Work out the finished part from the listing and answer in its coordinate system (mm). A direction names the side the tool comes from. Give positions to 0.01 mm unless a question says otherwise; leave off trailing zeros. Loops run counter-clockwise (first coordinate to the right, second up) from the corner with the lowest first, then second, coordinate; pieces in that order, holes last. Notation, with made-up numbers: M -7.75,-26 L 10.25,-26 A32 cw 10.25,3 Z; hole C 65.25,41.25 d3. An arc over 180 degrees is marked long. Use a Markdown table: item, result.
```python
from build123d import *

# Parameters (mm, degrees)
SKETCH_R              = 50
PAD_DEPTH             = 3
SKETCH004_R           = 5.2
POCKET001_DEPTH       = 3.001
POCKET002_DEPTH       = 3.001
SKETCH006_R           = 50
SKETCH006_R_2         = 46
PAD001_DEPTH          = 17.5
POCKET003_DEPTH       = 3
POLARPATTERN001_COUNT = 3
PAD002_DEPTH          = 2.8
POLARPATTERN002_COUNT = 3


with BuildPart() as part:
    # Sketch → Pad (new body)
    with BuildSketch(Plane.XY):
        Circle(SKETCH_R)
    extrude(amount=PAD_DEPTH)

    # Sketch004 (on DatumPlane) → Pocket001 (cut, through all)
    with BuildSketch(Plane.XY.offset(3)):
        Circle(SKETCH004_R)
    extrude(amount=-POCKET001_DEPTH, mode=Mode.SUBTRACT)

    # Sketch005 → Pocket002 (cut, through all)
    with BuildSketch(Plane.XY):
        with BuildLine():
            ThreePointArc((12.9390240745, -44.1427418269), (23, -39.8371685741), (31.7592237776, -33.2768944622))
            Line((16.9700186383, -18.3580627359), (31.7592237776, -33.2768944622))
            ThreePointArc((7.4135393744, -23.8754986114), (12.5, -21.6506350946), (16.9700186383, -18.3580627359))
            Line((12.9390240745, -44.1427418269), (7.4135393744, -23.8754986114))
        make_face()
    extrude(amount=POCKET002_DEPTH, mode=Mode.SUBTRACT)

    # Sketch006 → Pad001 (join)
    with BuildSketch(Plane.XY):
        Circle(SKETCH006_R)
        Circle(SKETCH006_R_2, mode=Mode.SUBTRACT)
    extrude(amount=-PAD001_DEPTH)

    # Sketch007 (on DatumPlane) → Pocket003 (cut)
    with BuildSketch(Plane.XY.offset(3)):
        with BuildLine():
            ThreePointArc((-45.3011566386, 7.9878161727), (-46, 0), (-45.3011566386, -7.9878161727))
            Line((-45.3011566386, -7.9878161727), (-47.2707721446, -8.335112528))
            ThreePointArc((-47.2707721446, 8.335112528), (-48, 0), (-47.2707721446, -8.335112528))
            Line((-47.2707721446, 8.335112528), (-45.3011566386, 7.9878161727))
        make_face()
    pocket003 = extrude(amount=-POCKET003_DEPTH, mode=Mode.SUBTRACT)

    # PolarPattern001: Pocket003 ×3 about axis
    polarpattern001_axis = Axis((0, 0, 3), (0, 0, 1))
    for i in range(1, POLARPATTERN001_COUNT):
        add(pocket003.rotate(polarpattern001_axis, i * 360 / POLARPATTERN001_COUNT), mode=Mode.SUBTRACT)

    # Sketch008 (on DatumPlane) → Pad002 (join)
    with BuildSketch(Plane.XY.offset(-17.5)):
        with BuildLine():
            ThreePointArc((45.3691376707, -7.5921898696), (46, 0), (45.3691376707, 7.5921898696))
            Line((47.1444517535, 7.8892755601), (45.3691376707, 7.5921898696))
            ThreePointArc((47.1444517535, -7.8892755601), (47.8, 0), (47.1444517535, 7.8892755601))
            Line((45.3691376707, -7.5921898696), (47.1444517535, -7.8892755601))
        make_face()
    pad002 = extrude(amount=-PAD002_DEPTH)

    # PolarPattern002: Pad002 ×3 about axis
    polarpattern002_axis = Axis((0, 0, -17.5), (0, 0, 1))
    for i in range(1, POLARPATTERN002_COUNT):
        add(pad002.rotate(polarpattern002_axis, i * 360 / POLARPATTERN002_COUNT))


solid = part.part
```
(1) Which of the six approach directions +Z, -Z, +X, -X, +Y, -Y give full straight-line access (tool end or side, diameter ignored) to faces 1 (the flat face through (10, 1, 0)), 2 (the cylindrical face through (23.898, -41.628, 1.521)), 3 (the flat face through (24.26, -25.71, 1.48))?
Entries:
| item | result |
|---|---|
| face 1 | -Z |
| face 2 | +Z |
| face 3 | +Z, -Z |
(2) Given P1, Ø10, axis at y = 27.5, z = -7, coming from the -X side; P2, Ø12, axis at x = -20, z = -7.5, coming from the -Y side; P3, Ø3, axis at x = 7, z = -6, coming from the +Y side, each flat-ended and moving along its own axis, determine where each tip first touches the part or whether it passes through.
Entries:
| item | result |
|---|---|
| P1 | stops at x = -44.65 |
| P2 | stops at y = -48 |
| P3 | stops at y = 49.7 |
(3) A cutting plane is placed at B-B (x = 0). Write down the section's boundary in (y, z), and give its area (3 significant figures).
Entries:
| item | result |
|---|---|
| outline | M -50,-17.5 L -46,-17.5 L -46,0 L -5.2,0 L -5.2,3 L -50,3 Z; M 5.2,0 L 46,0 L 46,-17.5 L 50,-17.5 L 50,3 L 5.2,3 Z |
| area | 409 mm² |
(4) The mould has two halves that part along Y. Classify faces 4 (the cylindrical face through (47.8, -0.1, -18.9)), 5 (the cylindrical face through (-23.804, 41.451, -18.88)), 6 (the flat face through (-47, 0, 0)), 7 (the cylindrical face through (-24, -41.34, -18.88)): released by +Y, released by -Y, zero draft, split by the parting line, or undercut.
Entries:
| item | result |
|---|---|
| face 4 | split by the parting line |
| face 5 | released by +Y |
| face 6 | undercut |
| face 7 | released by -Y |
(5) Consider probe 1 along Y at (x, z) = (0, 2.35); probe 2 along Y at (x, z) = (0, -11.75); probe 3 along X at (y, z) = (27.5, -11.5). Determine where each line is inside the solid, lowest interval first. Write a range as [from, to].
Entries:
| item | result |
|---|---|
| probe 1 | y = [-50, -5.2], [5.2, 50] |
| probe 2 | y = [-50, -46], [46, 50] |
| probe 3 | x = [-41.76, -36.87], [36.87, 41.76] |
(6) A cutting plane is placed at C-C (y = -27.5). Write down the section's boundary in (x, z).
Entries:
| item | result |
|---|---|
| outline | M -41.76,-17.5 L -36.87,-17.5 L -36.87,0 L 8.4,0 L 8.4,3 L -41.76,3 Z; M 26.03,0 L 36.87,0 L 36.87,-17.5 L 41.76,-17.5 L 41.76,3 L 26.03,3 Z |
